```python
from build123d import *

# Parameters (mm, degrees)
F4_R     = 9.525
F5_DEPTH = 29.36875
F6_R     = 9.525
F7_DEPTH = 29.36875
F8_R     = 9.525
F9_DEPTH = 29.36875


with BuildPart() as f1:
    # F0 (on Front) → F1 (revolve)
    with BuildSketch(Plane.XZ):
        with BuildLine():
            Line((0, 23.8125), (0, -23.8125))
            ThreePointArc((0, -23.8125), (23.8125, 0), (0, 23.8125))
        make_face()
    revolve(axis=Axis((0, 0, 0), (0, 0, -1)))

    # F2 (on Front) → F3 (revolve, cut)
    with BuildSketch(Plane.XZ):
        with BuildLine():
            Line((0, 14.28115), (0, -14.28115))
            ThreePointArc((0, -14.28115), (14.28115, 0), (0, 14.28115))
        make_face()
    revolve(axis=Axis((0, 0, 0), (0, 0, -1)), mode=Mode.SUBTRACT)

    # F4 (on Front) → F5 (cut, symmetric)
    with BuildSketch(Plane.XZ):
        Circle(F4_R)
    extrude(amount=F5_DEPTH, both=True, mode=Mode.SUBTRACT)

    # F6 (on Right) → F7 (cut, symmetric)
    with BuildSketch(Plane.YZ):
        Circle(F6_R)
    extrude(amount=F7_DEPTH, both=True, mode=Mode.SUBTRACT)

    # F8 (on Top) → F9 (cut, symmetric)
    with BuildSketch(Plane.XY):
        Circle(F8_R)
    extrude(amount=F9_DEPTH, both=True, mode=Mode.SUBTRACT)


solid = f1.part
```
The model under review builds one solid part; all positions refer to its coordinate system, in mm. Coordinates: 2 decimals unless noted, no trailing zeros. Write each loop counter-clockwise with the first axis right and the second up, starting at its lowest first coordinate (ties: lowest second). Pieces come first, ordered by that corner, then holes. Notation, with made-up numbers: (14.25, -3.5) - (41.25, -3.5) arc R14 cw to (41.25, 13.5) - close; hole circle Ø10 at (37, 8). An arc over 180 degrees is marked (long way). Write item = value, one per line.
(1) Consider section D-D, the plane x = 17. Give the boundary of the cut face in (y, z) (3 decimals).
Result sheet:
outline = circle Ø33.349 at (0, 0); hole circle Ø19.05 at (0, 0)
(2) Mouldability with a two-part tool opening along Z and no side actions: class faces 1 (the face through (-7.559, -5.796, 16.311)), 2 (the face through (-7.559, -16.311, -5.796)) as pulls with the +Z half, pulls with the -Z half, needs draft (parallel to the pull), parting line crosses it, or undercut.
Result sheet:
face_1 = needs draft
face_2 = undercut
(3) Consider section C-C, the plane z = -14. Give the boundary of the cut face in (x, y) (3 decimals), then the cut area to 3 significant figures.
Result sheet:
outline = circle Ø38.525 at (0, 0); hole circle Ø19.05 at (0, 0)
area = 881 mm^2
(4) Consider section A-A, the plane y = 0. Give the boundary of the cut face in (x, z) (1 decimal).
Result sheet:
outline = (-21.8, -9.5) arc R23.8 ccw to (-9.5, -21.8) - (-9.5, -10.6) arc R14.3 cw to (-10.6, -9.5) - close; (-21.8, 9.5) - (-10.6, 9.5) arc R14.3 cw to (-9.5, 10.6) - (-9.5, 21.8) arc R23.8 ccw to start; (9.5, -21.8) arc R23.8 ccw to (21.8, -9.5) - (10.6, -9.5) arc R14.3 cw to (9.5, -10.6) - close; (9.5, 10.6) arc R14.3 cw to (10.6, 9.5) - (21.8, 9.5) arc R23.8 ccw to (9.5, 21.8) - close
(5) For P1, Ø1, axis at x = -9, y = -15.5, coming from the -Z side; P2, Ø8, axis at x = 17.5, y = 8.5, coming from the -Z side; P3, Ø1.5, axis at y = 15.5, z = -10, coming from the +X side, all flat-tipped, find the tip position at first contact; note any pin that passes through.
Result sheet:
P1 = -16.23
P2 = -18.12
P3 = 15.93
(6) For line 1 (Y direction, x = -6, z = 9.5); line 2 (Z direction, x = 18.25, y = 0) (3 decimals); line 3 (Z direction, x = -2, y = 20.5), list the stretches that pass through material, from the lowest coordinate up. Write a range as [from, to].
Result sheet:
line_1 = [-20.99, -8.81], [8.81, 20.99]
line_2 = [-15.296, -9.525], [9.525, 15.296]
line_3 = [-11.95, -9.31], [9.31, 11.95]
